Autodesk Inventor part; units mm, degrees
ref_plane "YZ Plane" through (0, 0, 0) normal (1, 0, 0) x (0, 1, 0)
ref_plane "XZ Plane" through (0, 0, 0) normal (0, 1, 0) x (-1, 0, 0)
ref_plane "XY Plane" through (0, 0, 0) normal (0, 0, 1) x (1, 0, 0)
sketch "Sketch1" plane through (0, 0, 0) normal (0, 1, 0) x (-1, 0, 0)
  line L0 (110, -40) -> (-110, -40)
  line L1 (-110, -40) -> (-110, 40)
  line L2 (-110, 40) -> (110, 40)
  line L3 (110, 40) -> (110, -40)
  line L4 (0, -40) -> (0, 40) construction
  line L5 (110, 0) -> (-110, 0) construction
  circle A0 centre (13.5, 0) radius 2.5
  circle A1 centre (-13.5, 0) radius 2.5
  line L6 (46, -40) -> (46, 40) construction
  line L7 (61.25, -13) -> (30.75, -13) construction
  line L8 (30.75, -13) -> (30.75, 13) construction
  line L9 (30.75, 13) -> (61.25, 13) construction
  line L10 (61.25, 13) -> (61.25, -13) construction
  line L11 (46, 13) -> (46, -13) construction
  line L12 (61.25, 0) -> (30.75, 0) construction
  circle A2 centre (30.75, -13) radius 2.75
  circle A3 centre (61.25, -13) radius 2.75
  circle A4 centre (61.25, 13) radius 2.75
  circle A5 centre (30.75, 13) radius 2.75
  circle A6 centre (-30.75, -13) radius 2.75
  circle A7 centre (-61.25, -13) radius 2.75
  circle A8 centre (-61.25, 13) radius 2.75
  circle A9 centre (-30.75, 13) radius 2.75
  circle A10 centre (95, -25) radius 5
  circle A11 centre (13.5, 30) radius 1.6
  circle A12 centre (-13.5, 30) radius 1.6
  point P0 (0, 0)
  point P1 (0, 0)
  dimension "d0" = 220
  dimension "d1" = 80
  dimension "d2" = 5
  dimension "d3" = 27
  dimension "d4" = 92
  dimension "d5" = 30.5
  dimension "d6" = 26
  dimension "d7" = 5.5
  dimension "d8" = 5.5
  dimension "d9" = 5.5
  dimension "d10" = 5.5
  dimension "d19" = 10
  dimension "d20" = 15
  dimension "d21" = 3.2
  dimension "d22" = 27
  dimension "d23" = 10
  dimension "d44" = 15
extrude "Extrusion1" add sketch "Sketch1" along normal blind 20
sketch "Sketch2" plane through (0, 20, 0) normal (0, 1, 0) x (1, 0, 0)
  line L0 (110, 40) -> (-110, 40)
  line L1 (-15, 40) -> (15, 40)
  line L2 (15, 40) -> (15, 37)
  line L3 (15, 37) -> (-15, 37)
  line L4 (-15, 37) -> (-15, 40)
  line L5 (0, 37) -> (0, 40) construction
  line L6 (-110, -40) -> (110, -40) construction
  line L7 (0, -40) -> (0, 40) construction
  point P0 (0, 0)
  point P1 (15, 40)
  dimension "d26" = 30
  dimension "d27" = 3
extrude "Extrusion2" add sketch "Sketch2" along normal blind 30
sketch "Sketch3" plane through (0, 20, 0) normal (0, 1, 0) x (1, 0, 0)
  circle A0 centre (30.75, -13) radius 2.75
  circle A1 centre (61.25, -13) radius 2.75
  circle A2 centre (61.25, 13) radius 2.75
  circle A3 centre (30.75, 13) radius 2.75
  circle A4 centre (13.5, 0) radius 2.5
  circle A5 centre (13.5, -30) radius 1.6
  line L0 (-110, -40) -> (110, -40) construction
  line L1 (0, -40) -> (0, 40) construction
  line L2 (110, 40) -> (-110, 40) construction
  circle A6 centre (13.5, -30) radius 1.6
  circle A7 centre (13.5, -30) radius 3.5
  circle A8 centre (13.5, 0) radius 4.5
  circle A9 centre (30.75, -13) radius 4.5
  circle A10 centre (30.75, 13) radius 4.5
  circle A11 centre (61.25, -13) radius 4.5
  circle A12 centre (61.25, 13) radius 4.5
  circle A13 centre (-30.75, -13) radius 2.75
  circle A14 centre (-61.25, -13) radius 2.75
  circle A15 centre (-61.25, 13) radius 2.75
  circle A16 centre (-30.75, 13) radius 2.75
  circle A17 centre (-13.5, 0) radius 2.5
  circle A18 centre (-13.5, -30) radius 1.6
  circle A19 centre (-13.5, -30) radius 1.6
  circle A20 centre (-13.5, -30) radius 3.5
  circle A21 centre (-13.5, 0) radius 4.5
  circle A22 centre (-30.75, -13) radius 4.5
  circle A23 centre (-30.75, 13) radius 4.5
  circle A24 centre (-61.25, -13) radius 4.5
  circle A25 centre (-61.25, 13) radius 4.5
  point P0 (0, 0)
  dimension "d30" = 7
  dimension "d31" = 9
  dimension "d32" = 9
  dimension "d33" = 9
  dimension "d34" = 9
  dimension "d35" = 9
extrude "Extrusion3" cut sketch "Sketch3" against normal blind 10 contours A3 | A5 | A7 | A8 | A9 | A10 | A11 | A12 | A15 | A18 | A20 | A21 | A22 | A23 | A24 | A25
sketch "Sketch4" plane through (110, 0, 40) normal (1, 0, 0) x (0, 0, -1)
  line L0 (0, 0) -> (0, 20) construction
  line L1 (0, 10) -> (80, 10) construction
  line L2 (80, 0) -> (80, 20) construction
  line L3 (40, 0) -> (40, 20) construction
  line L4 (0, 20) -> (80, 20) construction
  circle A0 centre (10, 10) radius 3.5
  circle A1 centre (70, 10) radius 3.5
  dimension "d38" = 7
  dimension "d39" = 60
extrude "Extrusion4" cut sketch "Sketch4" against normal blind 11
sketch "Sketch5" plane through (-110, 0, -40) normal (-1, 0, 0) x (0, 0, 1)
  circle A0 centre (70, 10) radius 3.5
  circle A1 centre (10, 10) radius 3.5
  point P0 (40, 0)
extrude "Extrusion5" cut sketch "Sketch5" against normal blind 11
sketch "Sketch6" plane through (0, 20, 0) normal (0, 1, 0) x (1, 0, 0)
  circle A0 centre (-50, 30) radius 2.5
  line L0 (15, 40) -> (-15, 40)
  line L1 (0, 40) -> (0, 37) construction
  line L2 (15, 37) -> (-15, 37) construction
  point P0 (0, 0)
  dimension "d45" = 5
  dimension "d46" = 10
  dimension "d47" = 50
extrude "Extrusion6" cut sketch "Sketch6" against normal blind 5
properties part number "universal_mount"
The model under review builds one solid part; all positions refer to its coordinate system, in mm. A direction names the side the tool comes from. Coordinates: 2 decimals unless noted, no trailing zeros. Write each loop counter-clockwise with the first axis right and the second up, starting at its lowest first coordinate (ties: lowest second). Pieces come first, ordered by that corner, then holes.
1) To check wall thickness, follow probe 1 along Z at (x, y) = (61, 15); probe 2 along Z at (x, y) = (-13, 12); probe 3 along X at (y, z) = (15.5, 27). State the ranges of each line that lie inside material, in increasing order.
2) Clearance check with flat-ended pins moving along their axes: pin 1 Ø4 at (x, z) = (-13.5, 30) entering from +Y; pin 2 Ø5.5 at (y, z) = (10, 30) entering from -X; pin 3 Ø0.9 at (y, z) = (30, -38) entering from +X. State where each tip first meets the part, or that it passes through.
3) We need section A-A on y = 17.5. Count the separate pieces of the cut face and the enclosed holes in it, then the cut area to 3 significant figures.
4) Machinability: for faces 1 (the face through (64, 5, 13)), 2 (the face through (-56.958, 15.07, 11.648)), which of the approach directions +Z, -Z, +X, -X, +Y, -Y give a long, thin tool a straight path to every point of the face, cutting with its end or side? Answer none if there is none.
5) The part is to be moulded in two halves that separate along X. For faces 3 (the face through (-58.5, 4.9, 12.9)), 4 (the face through (-104.577, 6.895, 31.615)), 5 (the face through (-26.458, 15.07, 11.648)), 6 (the face through (-99, 10, -31)), say which applies: pulls with the +X half, pulls with the -X half, needs draft (parallel to the pull), parting line crosses it, or undercut.
6) We need section B-B on z = 0. State the section outline as (x, y) points, then the cut area to 3 significant figures.
7) We need section C-C on x = -96.5. State the section outline as (y, z) points.
Answer list:
1. probe 1: z = -40 to -17.49, -8.51 to 8.51, 17.49 to 40
1. probe 2: z = -40 to -4.47, 4.47 to 26.54, 33.46 to 40
1. probe 3: x = -110 to -15.3, -11.7 to 11.7, 15.3 to 110
2. pin 1: stops at y = 10
2. pin 2: stops at x = -99
2. pin 3: stops at x = 15
3. separate pieces: 1
3. enclosed holes: 14
3. area: 16,800 mm2
4. face 1: +Y, -Y
4. face 2: +Y
5. face 3: undercut
5. face 4: needs draft
5. face 5: undercut
5. face 6: pulls with the -X half
6. outline: (-110, 0) - (-16, 0) - (-16, 10) - (-18, 10) - (-18, 20) - (-110, 20) - close; (-11, 0) - (11, 0) - (11, 10) - (9, 10) - (9, 20) - (-9, 20) - (-9, 10) - (-11, 10) - close; (16, 0) - (110, 0) - (110, 20) - (18, 20) - (18, 10) - (16, 10) - close
6. area: 4,120 mm2
7. outline: (0, -40) - (20, -40) - (20, -29.77) - (0, -29.77) - close; (0, -20.23) - (20, -20.23) - (20, 40) - (0, 40) - close
